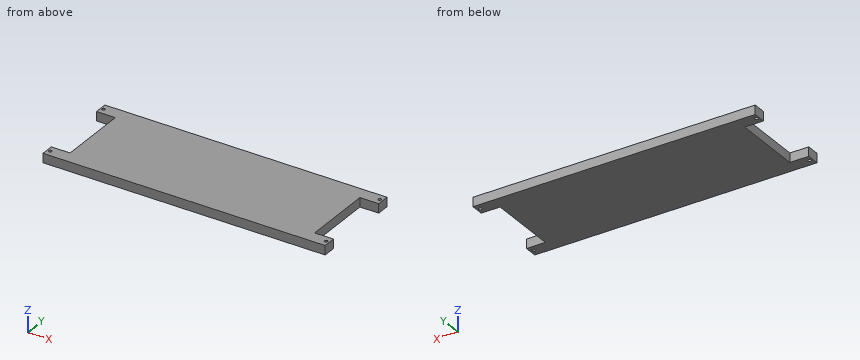
```python
from build123d import *

# Parameters (mm, degrees)
F1_DEPTH = 4.9
F2_R     = 0.85
F3_DEPTH = 4.901


with BuildPart() as f1:
    # F0 (on Top) → F1 (new body)
    with BuildSketch(Plane.XY):
        Polygon((-75, -25.4), (75, -25.4), (75, -18.6), (65, -18.6), (65, 18.6), (75, 18.6), (75, 25.4), (-75, 25.4), (-75, 18.6), (-65, 18.6), (-65, -18.6), (-75, -18.6), align=None)
    extrude(amount=F1_DEPTH)

    # F2 (on face) → F3 (cut, through all)
    with BuildSketch(Plane.XY.offset(4.9)):
        with Locations((-73.5, 22)):
            Circle(F2_R)
        with Locations((-73.3, -22)):
            Circle(F2_R)
        with Locations((73.3, 22)):
            Circle(F2_R)
        with Locations((73.3, -22)):
            Circle(F2_R)
    extrude(amount=-F3_DEPTH, mode=Mode.SUBTRACT)


solid = f1.part
```
Read the model definition and answer for the solid it produces. Units are mm, in the model's axes. Give positions to 0.01 mm unless a question says otherwise; leave off trailing zeros. Write each loop counter-clockwise with the first axis right and the second up, starting at its lowest first coordinate (ties: lowest second). Pieces come first, ordered by that corner, then holes. Notation, with made-up numbers: M 69.25,-13.5 L 121.25,-13.5 A25 cw 121.25,22.5 Z; hole C 63,58.25 d5. An arc over 180 degrees is marked long. Put each result on its own line as item: value. Start each with the question number.
1. The part is cut by section B-B, the plane y = -8.5. Give the vertices of the cut face in (x, z).
2. The part is cut by section A-A, the plane z = 2.35. Give the vertices of the cut face in (x, y), and give its area (3 significant figures).
3. This flat-tipped pin is pushed along its axis until it touches: pin 1 Ø2.5 at (y, z) = (1, 2.5) entering from +X. Where does it stop, or does it pass through?
4. Consider line 1 along Y through (x, z) = (73.3, 2.55); line 2 along X through (y, z) = (-18.5, 2.9); line 3 along X through (y, z) = (22.5, 0.9). Determine where each line is inside the solid, lowest interval first.
Final values:
1. outline: M -65,0 L 65,0 L 65,4.9 L -65,4.9 Z
2. outline: M -75,-25.4 L 75,-25.4 L 75,-18.6 L 65,-18.6 L 65,18.6 L 75,18.6 L 75,25.4 L -75,25.4 L -75,18.6 L -65,18.6 L -65,-18.6 L -75,-18.6 Z; hole C -73.5,22 d1.7; hole C -73.3,-22 d1.7; hole C 73.3,-22 d1.7; hole C 73.3,22 d1.7
2. area: 6,870 mm²
3. pin 1: stops at x = 65
4. line 1: y = -25.4 to -22.85, -21.15 to -18.6, 18.6 to 21.15, 22.85 to 25.4
4. line 2: x = -65 to 65
4. line 3: x = -75 to -74.19, -72.81 to 72.61, 73.99 to 75
